```python
from build123d import *

# Parameters (mm, degrees)
F0_W      = 28
F0_H      = 30
F1_DEPTH  = 4
F2_R      = 6.25
F2_W      = 6
F2_H      = 23
F2_W_2    = 16.817460835
F2_H_2    = 13.5
F3_DEPTH  = 25
F4_W      = 6
F4_H      = 7
F4_R      = 6.25
F5_DEPTH  = 5
F6_DEPTH  = 17
F8_DEPTH  = 25
F9_R      = 5
F10_R     = 3
F11_R     = 5
F12_DEPTH = 2


with BuildPart() as f1:
    # F0 (on Top) → F1 (new body)
    with BuildSketch(Plane.XY):
        with Locations((14, 15)):
            Rectangle(F0_W, F0_H)
    extrude(amount=F1_DEPTH)

    # F2 (on face) → F3 (cut)
    with BuildSketch(Plane.XY.offset(4)):
        with Locations((16.75, 21.75)):
            Circle(F2_R)
        with Locations((3, 18.5)):
            Rectangle(F2_W, F2_H)
        with Locations((19.5912695825, 6.75)):
            Rectangle(F2_W_2, F2_H_2)
    extrude(amount=-F3_DEPTH, mode=Mode.SUBTRACT)

    # F4 (on face) → F5 (join)
    with BuildSketch(Plane.XY.offset(4)):
        with Locations((3, 3.5)):
            Rectangle(F4_W, F4_H)
        Polygon((6, 30), (6, 7), (6, 0), (11.182539165, 0), (11.182539165, 13.5), (28, 13.5), (28, 30), align=None)
        with Locations((16.75, 21.75)):
            Circle(F4_R, mode=Mode.SUBTRACT)
    extrude(amount=F5_DEPTH)

    # F4 (on face) → F6 (join)
    with BuildSketch(Plane.XY.offset(4)):
        with Locations((3, 3.5)):
            Rectangle(F4_W, F4_H)
    extrude(amount=F6_DEPTH)

    # F7 (on face) → F8 (cut)
    with BuildSketch(Plane.XZ):
        with BuildLine():
            ThreePointArc((3.6420098484, 3), (3.1733806983, 4.1313708499), (2.0420098484, 4.6))
            ThreePointArc((2.0420098484, 4.6), (0.9106389985, 1.8686291501), (3.6420098484, 3))
        make_face()
        with BuildLine():
            ThreePointArc((3.6420098484, 18), (0.9106389985, 19.1313708499), (2.0420098484, 16.4))
            ThreePointArc((2.0420098484, 16.4), (3.1733806983, 16.8686291501), (3.6420098484, 18))
        make_face()
    extrude(amount=-F8_DEPTH, mode=Mode.SUBTRACT)

    # F9
    f9_edges = [f1.edges().sort_by_distance(p)[0] for p in [
        (28, 13.5, 4.5),
        (28, 30, 4.5),
        (6, 30, 4.5),
    ]]
    fillet(f9_edges, radius=F9_R)

    # F10
    f10_edges = [f1.edges().sort_by_distance(p)[0] for p in [
        (11.182539, 13.5, 4.5),
    ]]
    fillet(f10_edges, radius=F10_R)

    # F11
    f11_edges = [f1.edges().sort_by_distance(p)[0] for p in [
        (6, 3.5, 9),
    ]]
    fillet(f11_edges, radius=F11_R)

    # F12 (add): a face of the model
    f12_faces = [f1.faces().sort_by_distance(p)[0] for p in [
        (0, 3.5, 10.5),
    ]]
    extrude(f12_faces, amount=F12_DEPTH)


solid = f1.part
```
CAD build for the part. Positions are in the model's coordinates, mm. A direction names the side the tool comes from. Round coordinates to 2 decimals unless told otherwise and drop trailing zeros. Loops run counter-clockwise (first coordinate to the right, second up) from the corner with the lowest first, then second, coordinate; pieces in that order, holes last. Notation, with made-up numbers: M 29.25,49.25 L 66.25,49.25 A23 cw 66.25,66.25 Z; hole C 72,-20.75 d5. An arc over 180 degrees is marked long. Use a Markdown table: item, result. Add a question column.
(1) Drill centre lines: line 1 (X direction, y = 4, z = 18); line 2 (X direction, y = 5.5, z = 3); line 3 (Z direction, x = 3.5, y = 4). Where is each one in solid material? Low to high.
(2) Cut at C-C (x = 3). Give the cut face in (y, z).
(3) Flat gauge pins, fed straight in: pin 1 (4 mm diameter, centred on x = 3, z = 9.5, fed in from +Y); pin 2 (6 mm diameter, centred on x = 11.5, y = 21, fed in from -Z); pin 3 (1.5 mm diameter, centred on y = 27, z = 5, fed in from -X); pin 4 (3 mm diameter, centred on y = 13, z = 4, fed in from +X). Where does each tip first touch, or does it go through?
(4) Which spindle directions (+Z, -Z, +X, -X, +Y, -Y) get a long thin tool onto all of the face, cutting with end or side? Do faces 1 (the face through (-2, 3, 10)), 2 (the face through (6, 16, 4)), 3 (the face through (6, 3, 17)), 4 (the face through (11.183, 5, 4)). Say none if no direction does.
(5) Cut at B-B (y = 21.75). Give the cut face in (x, z), and give its area (3 significant figures).
(6) Cut at A-A (x = 16.75). Give the cut face in (y, z).
(7) Cut at D-D (y = 9.5). Give the cut face in (x, z), and give its area (3 significant figures).
Geometry says:
| question | item | result |
|---|---|---|
| 1 | line 1 | x = -2 to 0.44, 3.64 to 6 |
| 1 | line 2 | x = -2 to 0.44, 3.64 to 11.18 |
| 1 | line 3 | z = 0 to 2.34, 3.66 to 17.34, 18.66 to 21 |
| 2 | outline | M 0,0 L 7,0 L 7,1.72 L 0,1.72 Z; M 0,4.28 L 7,4.28 L 7,16.72 L 0,16.72 Z; M 0,19.28 L 7,19.28 L 7,21 L 0,21 Z |
| 3 | pin 1 | stops at y = 7 |
| 3 | pin 2 | stops at z = 0 |
| 3 | pin 3 | stops at x = 6.16 |
| 3 | pin 4 | stops at x = 26 |
| 4 | face 1 | +Z, -Z, -X, +Y, -Y |
| 4 | face 2 | +Z, -Z, -X, +Y |
| 4 | face 3 | +Z, +X, +Y, -Y |
| 4 | face 4 | +Z, -Z, +X, -Y |
| 5 | outline | M 6,0 L 10.5,0 L 10.5,9 L 6,9 Z; M 23,0 L 28,0 L 28,9 L 23,9 Z |
| 5 | area | 85.5 mm² |
| 6 | outline | M 13.5,0 L 15.5,0 L 15.5,9 L 13.5,9 Z; M 28,0 L 30,0 L 30,9 L 28,9 Z |
| 7 | outline | M 6,0 L 11.18,0 L 11.18,9 L 6,9 Z |
| 7 | area | 46.6 mm² |
